```python
from build123d import *

# Parameters (mm, degrees)
EXTRUDE_1_DEPTH     = 35
CUT_EXTRUDE_1_DEPTH = 17


with BuildPart() as part:
    # 草圖1 → 填料-伸長1 (new body)
    with BuildSketch(Plane.XY):
        Polygon((-6.958874233, 13), (-6.958874233, 0), (6.041125767, 0), (6.041125767, 13), (13, 13), (13, -13), (6.041125767, -13), (6.041125767, -6), (-6.958874233, -6), (-6.958874233, -13), (-13, -13), (-13, 13), align=None)
    extrude(amount=EXTRUDE_1_DEPTH)

    # 草圖2 → 除料-伸長1 (cut)
    with BuildSketch(Plane(origin=(0, 13, 0), x_dir=(1, 0, 0), z_dir=(0, 1, 0))):
        Polygon((13, -35), (-6.958874233, -13.50582775), (-6.958874233, -35), align=None)
        Polygon((-6.958874233, -13.50582775), (-13, -7), (-13, -35), (-6.958874233, -35), align=None)
    extrude(amount=-CUT_EXTRUDE_1_DEPTH, mode=Mode.SUBTRACT)


solid = part.part
```
Check sheet for the modelled part. Datum: model origin and axes. Units: mm. A direction names the side the tool comes from. Give positions to 0.01 mm unless a question says otherwise; leave off trailing zeros. Write each loop counter-clockwise with the first axis right and the second up, starting at its lowest first coordinate (ties: lowest second). Pieces come first, ordered by that corner, then holes. Notation, with made-up numbers: (41.5, 9) - (55.5, 9) arc R33 cw to (55.5, 46) - close; hole circle Ø8 at (23.25, -23.75). An arc over 180 degrees is marked (long way). Answer as a JSON object with one key per item and string values. Group by question number.
1) Release check for a two-part mould opening along X. For faces 1 (the face through (-10, -13, 17)), 2 (the face through (-13, -6, 13)), 3 (the face through (-1, 0, 11)) record: pulls with the +X half, pulls with the -X half, needs draft (parallel to the pull), parting line crosses it, or undercut.
2) Depth check by flat-ended pin: P1, Ø1.5, axis at y = 7.5, z = 10.5, coming from the -X side; P2, Ø14.5, axis at y = 4, z = 20.5, coming from the -X side; P3, Ø8, axis at x = 6, y = 5, coming from the +Z side. Enter the tip coordinate at first touch or a pass-through.
3) Thickness scan on probe 1 along X at (y, z) = (-9.75, 4); probe 2 along Y at (x, z) = (-4.5, 32); probe 3 along X at (y, z) = (11.25, 26). Record the ranges inside material, lowest first. Write a range as from..to.
4) Sectioned sample at B-B (z = 6.5). Record the cut outline in (x, y).
5) Sectioned sample at C-C (y = -11). Record the cut outline in (x, z), then the cut area to 3 significant figures.
6) Sectioned sample at A-A (y = 2.5). Record the cut outline in (x, z), then the cut area to 3 significant figures.
7) Access from +Z, -Z, +X, -X, +Y, -Y to the whole of each face (thin tool, end or side, straight path). Record for faces 4 (the face through (-6, -4, 27)), 5 (the face through (-6.959, 7, 7)), 6 (the face through (-6.959, -9, 17)).
8) Sectioned sample at D-D (x = 11). Record the cut outline in (y, z), then the cut area to 3 significant figures.
Geometry results:
{
 "1": {"face 1": "needs draft", "face 2": "pulls with the -X half", "face 3": "undercut"},
 "2": {"P1": "stops at x = -10.45", "P2": "stops at x = -7.2", "P3": "stops at z = 31.77"},
 "3": {"probe 1": "x = -13..-6.96, 6.04..13", "probe 2": "y = -6..-4", "probe 3": "x = 6.04..13"},
 "4": {"outline": "(-13, -13) - (-6.96, -13) - (-6.96, -6) - (6.04, -6) - (6.04, -13) - (13, -13) - (13, 13) - (6.04, 13) - (6.04, 0) - (-6.96, 0) - (-6.96, 13) - (-13, 13) - close"},
 "5": {"outline": "(-13, 0) - (-6.96, 0) - (-6.96, 35) - (-13, 35) - close; (6.04, 0) - (13, 0) - (13, 35) - (6.04, 35) - close", "area": "455 mm^2"},
 "6": {"outline": "(-13, 0) - (-6.96, 0) - (-6.96, 13.51) - (-13, 7) - close; (6.04, 0) - (13, 0) - (13, 35) - (6.04, 27.51) - close", "area": "279 mm^2"},
 "7": {"face 4": "+Z, -X, +Y", "face 5": "+Z, -Z, +Y", "face 6": "+Z, -Z, -Y"},
 "8": {"outline": "(-13, 0) - (13, 0) - (13, 32.85) - (-4, 32.85) - (-4, 35) - (-13, 35) - close", "area": "873 mm^2"}
}
